Model file for the job. Use its own axes, mm. A direction names the side the tool comes from. Give positions to 0.01 mm unless a question says otherwise; leave off trailing zeros. Order: outer loops, then holes, each group sorted by start corner. A loop starts at its lowest first (then second) coordinate and runs counter-clockwise, first axis right, second up. Notation, with made-up numbers: M 59,-7 L 89,-7 A15 cw 89,7 Z; hole C 66,-7 d1. An arc over 180 degrees is marked long. Return JSON: item names as keys, results as strings. Group by question number.
1. Slice it at D-D on z = -8.75. List the corners of the cut face in (x, y).
2. Slice it at B-B on z = -17.5. List the corners of the cut face in (x, y), then the cut area to 3 significant figures.
3. Wall check: probe 1 along X at (y, z) = (-36.5, -7.5); probe 2 along Y at (x, z) = (2, -14.75); probe 3 along Y at (x, z) = (-20.5, -8). Give the ranges that are in metal, low to high. Write a range as [from, to].
4. Two-plate mould, pull along X, no slides. Class faces 4 (the face through (-42, 1, 4)), 5 (the face through (-22, 29, -5)), 6 (the face through (41.787, 41.748, -10.195)), 7 (the face through (39, -35.7, -18)): released by +X, released by -X, zero draft, split by the parting line, or undercut.
5. Slice it at C-C on x = -5. List the corners of the cut face in (y, z), then the cut area to 3 significant figures.
6. Pin check, flat tips, straight feed: pin 1 (10 mm diameter, centred on x = -11, y = -25, fed in from -Z); pin 2 (1.4 mm diameter, centred on x = -34.48, y = 11.2, fed in from -Z); pin 3 (2 mm diameter, centred on x = 40.5, z = -14.5, fed in from -Y); pin 4 (1.7 mm diameter, centred on x = 21.31, y = 29.33, fed in from +Z). Stop position of each tip, or through.
7. 3-axis set-ups, long thin cutter, end or side, ignore diameter. For faces 1 (the face through (41, -24, -15.75)), 2 (the face through (25.75, 28, -12)), 3 (the face through (0.29, 37.73, -5.98)): which of +Z, -Z, +X, -X, +Y, -Y reach the whole face in a straight line?
8. Slice it at A-A on y = 14. List the corners of the cut face in (x, z), then the cut area to 3 significant figures.
from build123d import *

# Parameters (mm, degrees)
ESQUISSE1_W                  = 85
ESQUISSE1_H                  = 85
BOSS_EXTRU_1_DEPTH           = 5
ESQUISSE2_R                  = 30.5
ENL_V_MAT_EXTRU_1_DEPTH      = 6
BOSS_EXTRU_2_DEPTH           = 3
ESQUISSE4_W                  = 85
ESQUISSE4_H                  = 85
BOSS_EXTRU_4_DEPTH           = 10
ESQUISSE5_W                  = 85
ESQUISSE5_H                  = 85
BOSS_EXTRU_5_DEPTH           = 3.25
ESQUISSE6_R                  = 39.5
ESQUISSE6_R_2                = 33
ENL_V_MAT_EXTRU_2_DEPTH      = 3.5
ESQUISSE7_R                  = 2.25
ENL_V_MAT_EXTRU_3_DEPTH      = 14.75
ESQUISSE8_W                  = 85
ESQUISSE8_H                  = 85
BOSS_EXTRU_6_DEPTH           = 10
CONG_1_R                     = 2.5
ESQUISSE9_W                  = 41.5
ESQUISSE9_H                  = 9
ENL_V_MAT_EXTRU_4_DEPTH      = 13.25
ESQUISSE10_R                 = 0.75
ENL_V_MAT_EXTRU_5_DEPTH      = 1
ESQUISSE11_R                 = 1.5
ENL_V_MAT_EXTRU_6_DEPTH      = 23.25
ENL_V_MAT_EXTRU_7_DEPTH      = 83.5
ENL_V_MAT_EXTRU_7_DEPTH_BACK = 3.5


with BuildPart() as part:
    # Esquisse1 → Boss.-Extru.1 (new body)
    with BuildSketch(Plane.XY):
        Rectangle(ESQUISSE1_W, ESQUISSE1_H)
    extrude(amount=BOSS_EXTRU_1_DEPTH)

    # Esquisse2 → Enlèv. mat.-Extru.1 (cut, through all)
    with BuildSketch(Plane.XY.offset(5)):
        Circle(ESQUISSE2_R)
    extrude(amount=-ENL_V_MAT_EXTRU_1_DEPTH, mode=Mode.SUBTRACT)

    # Esquisse3 → Boss.-Extru.2 (add)
    with BuildSketch(Plane(origin=(0, 0, 0), x_dir=(-1, 0, 0), z_dir=(0, 0, -1))):
        with BuildLine():
            Line((-32.337091706, 3.25), (-42.5, 3.25))
            Line((-42.5, 3.25), (-42.5, -3.25))
            Line((-42.5, -3.25), (-32.337091706, -3.25))
            ThreePointArc((-32.337091706, -3.25), (-32.5, 0), (-32.337091706, 3.25))
        make_face()
        with BuildLine():
            Line((32.337091706, -3.25), (42.5, -3.25))
            Line((42.5, -3.25), (42.5, 3.25))
            Line((42.5, 3.25), (32.337091706, 3.25))
            ThreePointArc((32.337091706, 3.25), (32.5, 0), (32.337091706, -3.25))
        make_face()
    extrude(amount=BOSS_EXTRU_2_DEPTH)

    # Esquisse4 → Boss.-Extru.4 (add)
    with BuildSketch(Plane(origin=(0, 0, 0), x_dir=(-1, 0, 0), z_dir=(0, 0, -1))):
        Rectangle(ESQUISSE4_W, ESQUISSE4_H)
        with BuildLine():
            Line((-23.5, 29), (-20.475595229, 29))
            ThreePointArc((-20.475595229, 29), (0, 35.5), (20.475595229, 29))
            Line((20.475595229, 29), (23.5, 29))
            Line((23.5, 29), (23.5, 26.608269391))
            ThreePointArc((23.5, 26.608269391), (32.996010976, 13.096307101), (35.350919366, -3.25))
            ThreePointArc((35.350919366, -3.25), (31.658488037, -16.062071324), (23.5, -26.608269391))
            Line((23.5, -26.608269391), (23.5, -29))
            Line((23.5, -29), (20.475595229, -29))
            ThreePointArc((20.475595229, -29), (0, -35.5), (-20.475595229, -29))
            Line((-20.475595229, -29), (-23.5, -29))
            Line((-23.5, -29), (-23.5, -26.608269391))
            ThreePointArc((-23.5, -26.608269391), (-31.658488037, -16.062071324), (-35.350919366, -3.25))
            ThreePointArc((-35.350919366, -3.25), (-32.996010976, 13.096307101), (-23.5, 26.608269391))
            Line((-23.5, 26.608269391), (-23.5, 29))
        make_face(mode=Mode.SUBTRACT)
    extrude(amount=BOSS_EXTRU_4_DEPTH)

    # Esquisse5 → Boss.-Extru.5 (add)
    with BuildSketch(Plane(origin=(0, 0, -10), x_dir=(-1, 0, 0), z_dir=(0, 0, -1))):
        Rectangle(ESQUISSE5_W, ESQUISSE5_H)
        with BuildLine():
            Line((14.838716252, 32.25), (25.75, 32.25))
            Line((25.75, 32.25), (25.75, 24.437420077))
            ThreePointArc((25.75, 24.437420077), (35.5, 0), (25.75, -24.437420077))
            Line((25.75, -24.437420077), (25.75, -32.25))
            Line((25.75, -32.25), (14.838716252, -32.25))
            ThreePointArc((14.838716252, -32.25), (0, -35.5), (-14.838716252, -32.25))
            Line((-14.838716252, -32.25), (-25.75, -32.25))
            Line((-25.75, -32.25), (-25.75, -24.437420077))
            ThreePointArc((-25.75, -24.437420077), (-35.5, 0), (-25.75, 24.437420077))
            Line((-25.75, 24.437420077), (-25.75, 32.25))
            Line((-25.75, 32.25), (-14.838716252, 32.25))
            ThreePointArc((-14.838716252, 32.25), (0, 35.5), (14.838716252, 32.25))
        make_face(mode=Mode.SUBTRACT)
    extrude(amount=BOSS_EXTRU_5_DEPTH)

    # Esquisse6 → Enlèv. mat.-Extru.2 (cut)
    with BuildSketch(Plane.XY.offset(5)):
        Circle(ESQUISSE6_R)
        Circle(ESQUISSE6_R_2, mode=Mode.SUBTRACT)
    extrude(amount=-ENL_V_MAT_EXTRU_2_DEPTH, mode=Mode.SUBTRACT)

    # Esquisse7 → Enlèv. mat.-Extru.3 (cut)
    with BuildSketch(Plane(origin=(0, 0, -13.25), x_dir=(-1, 0, 0), z_dir=(0, 0, -1))):
        with Locations((0, 35.5)):
            Circle(ESQUISSE7_R)
    extrude(amount=-ENL_V_MAT_EXTRU_3_DEPTH, mode=Mode.SUBTRACT)

    # Esquisse8 → Boss.-Extru.6 (add)
    with BuildSketch(Plane(origin=(0, 0, -13.25), x_dir=(-1, 0, 0), z_dir=(0, 0, -1))):
        Rectangle(ESQUISSE8_W, ESQUISSE8_H)
        with BuildLine():
            Line((-25, 40), (25, 40))
            ThreePointArc((25, 40), (35.606601718, 35.606601718), (40, 25))
            Line((40, 25), (40, -25))
            ThreePointArc((40, -25), (35.606601718, -35.606601718), (25, -40))
            Line((25, -40), (-25, -40))
            ThreePointArc((-25, -40), (-35.606601718, -35.606601718), (-40, -25))
            Line((-40, -25), (-40, 25))
            ThreePointArc((-40, 25), (-35.606601718, 35.606601718), (-25, 40))
        make_face(mode=Mode.SUBTRACT)
    extrude(amount=BOSS_EXTRU_6_DEPTH)

    # Congé1
    cong_1_edges = [part.edges().sort_by_distance(p)[0] for p in [
        (-42.5, 0, 5),
        (0, -42.5, 5),
        (42.5, 0, 5),
        (42.5, -42.5, -9.125),
        (-42.5, -42.5, -9.125),
        (-42.5, 42.5, -9.125),
        (42.5, 42.5, -9.125),
        (0, 42.5, 5),
    ]]
    fillet(cong_1_edges, radius=CONG_1_R)

    # Esquisse9 → Enlèv. mat.-Extru.4 (cut)
    with BuildSketch(Plane(origin=(0, 0, -13.25), x_dir=(-1, 0, 0), z_dir=(0, 0, -1))):
        with Locations((0, -33.5)):
            Rectangle(ESQUISSE9_W, ESQUISSE9_H)
    extrude(amount=-ENL_V_MAT_EXTRU_4_DEPTH, mode=Mode.SUBTRACT)

    # Esquisse10 → Enlèv. mat.-Extru.5 (cut)
    with BuildSketch(Plane.XY.offset(1.5)):
        with Locations((0, 36.25)):
            Circle(ESQUISSE10_R)
        with Locations((21.307215396, 29.326866046)):
            Circle(ESQUISSE10_R)
        with Locations((34.475798716, 11.201866046)):
            Circle(ESQUISSE10_R)
        with Locations((34.475798716, -11.201866046)):
            Circle(ESQUISSE10_R)
        with Locations((21.307215396, -29.326866046)):
            Circle(ESQUISSE10_R)
        with Locations((0, -36.25)):
            Circle(ESQUISSE10_R)
        with Locations((-21.307215396, -29.326866046)):
            Circle(ESQUISSE10_R)
        with Locations((-34.475798716, -11.201866046)):
            Circle(ESQUISSE10_R)
        with Locations((-34.475798716, 11.201866046)):
            Circle(ESQUISSE10_R)
        with Locations((-21.307215396, 29.326866046)):
            Circle(ESQUISSE10_R)
    extrude(amount=-ENL_V_MAT_EXTRU_5_DEPTH, mode=Mode.SUBTRACT)

    # Esquisse11 → Enlèv. mat.-Extru.6 (cut)
    with BuildSketch(Plane(origin=(0, 0, -23.25), x_dir=(-1, 0, 0), z_dir=(0, 0, -1))):
        with Locations((38.687184335, 38.687184335)):
            Circle(ESQUISSE11_R)
        with Locations((38.687184335, -38.687184335)):
            Circle(ESQUISSE11_R)
        with Locations((-38.687184335, -38.687184335)):
            Circle(ESQUISSE11_R)
        with Locations((-38.687184335, 38.687184335)):
            Circle(ESQUISSE11_R)
    extrude(amount=-ENL_V_MAT_EXTRU_6_DEPTH, mode=Mode.SUBTRACT)

    # Esquisse12 → Enlèv. mat.-Extru.7 (cut, two sides)
    with BuildSketch(Plane.ZY.offset(-40)) as enl_v_mat_extru_7_sk:
        Polygon((-13.25, -21.4), (-15.75, -21.4), (-15.75, -25.7), (-19.25, -25.7), (-19.25, -35.7), (-15.75, -35.7), (-15.75, -40), (-13.25, -40), align=None)
    extrude(amount=ENL_V_MAT_EXTRU_7_DEPTH, mode=Mode.SUBTRACT)
    extrude(enl_v_mat_extru_7_sk.sketch, amount=-ENL_V_MAT_EXTRU_7_DEPTH_BACK, mode=Mode.SUBTRACT)


solid = part.part
Result:
{
 "1": {"outline": "M -42.5,-40 A2.5 ccw -40,-42.5 L 40,-42.5 A2.5 ccw 42.5,-40 L 42.5,40 A2.5 ccw 40,42.5 L -40,42.5 A2.5 ccw -42.5,40 Z; hole C -38.69,-38.69 d3; hole C -38.69,38.69 d3; hole M -23.5,-29 L -20.75,-29 L -20.75,-38 L 20.75,-38 L 20.75,-29 L 23.5,-29 L 23.5,-26.61 A35.5 ccw 23.5,26.61 L 23.5,29 L 20.48,29 A35.5 ccw 2.25,35.43 A2.25 ccw long -2.25,35.43 A35.5 ccw -20.48,29 L -23.5,29 L -23.5,26.61 A35.5 ccw -23.5,-26.61 Z; hole C 38.69,-38.69 d3; hole C 38.69,38.69 d3"},
 "2": {"outline": "M -42.5,-40 A2.5 ccw -40,-42.5 L 40,-42.5 A2.5 ccw 42.5,-40 L 42.5,-35.7 L 35.51,-35.7 A15 cw 25,-40 L -25,-40 A15 cw -35.51,-35.7 L -42.5,-35.7 Z; M -42.5,-25.7 L -39.98,-25.7 A15 cw -40,-25 L -40,25 A15 cw -25,40 L 25,40 A15 cw 40,25 L 40,-25 A15 cw 39.98,-25.7 L 42.5,-25.7 L 42.5,40 A2.5 ccw 40,42.5 L -40,42.5 A2.5 ccw -42.5,40 Z; hole C -38.69,-38.69 d3; hole C -38.69,38.69 d3; hole C 38.69,-38.69 d3; hole C 38.69,38.69 d3", "area": "905 mm2"},
 "3": {"probe 1": "x = [-42.5, -20.75], [20.75, 42.5]", "probe 2": "y = [-42.5, -40], [40, 42.5]", "probe 3": "y = [-42.5, -38], [29, 42.5]"},
 "4": {"face 4": "released by -X", "face 5": "undercut", "face 6": "released by +X", "face 7": "zero draft"},
 "5": {"outline": "M -42.5,-23.25 L -40,-23.25 L -40,-13.25 L -38,-13.25 L -38,0 L -30.09,0 L -30.09,5 L -32.62,5 L -32.62,1.5 L -39.18,1.5 L -39.18,5 L -40,5 A2.5 ccw -42.5,2.5 Z; M 30.09,0 L 35.15,0 L 35.15,-13.25 L 40,-13.25 L 40,-23.25 L 42.5,-23.25 L 42.5,2.5 A2.5 ccw 40,5 L 39.18,5 L 39.18,1.5 L 32.62,1.5 L 32.62,5 L 30.09,5 Z", "area": "283 mm2"},
 "6": {"pin 1": "stops at z = 0", "pin 2": "stops at z = -13.25", "pin 3": "stops at y = -42.5", "pin 4": "stops at z = 1.5"},
 "7": {"face 1": "+X, -X", "face 2": "-Z", "face 3": "+Z, -Z"},
 "8": {"outline": "M -42.5,-23.25 L -40,-23.25 L -40,-13.25 L -32.62,-13.25 L -32.62,0 L -27.1,0 L -27.1,5 L -29.88,5 L -29.88,1.5 L -36.94,1.5 L -36.94,5 L -40,5 A2.5 ccw -42.5,2.5 Z; M 27.1,0 L 32.62,0 L 32.62,-13.25 L 40,-13.25 L 40,-23.25 L 42.5,-23.25 L 42.5,2.5 A2.5 ccw 40,5 L 36.94,5 L 36.94,1.5 L 29.88,1.5 L 29.88,5 L 27.1,5 Z", "area": "414 mm2"}
}
